Design review of the part built by this model. Coordinates are the model's own, in mm. Give positions to 0.01 mm unless a question says otherwise; leave off trailing zeros. Loops run counter-clockwise (first coordinate to the right, second up) from the corner with the lowest first, then second, coordinate; pieces in that order, holes last. Notation, with made-up numbers: (74, 71.25) -> (93, 71.25) arc R24 cw to (93, 101.25) -> close; hole circle Ø10 at (67.25, 40). An arc over 180 degrees is marked (long way). Answer as CSV lines item,"result".
from build123d import *

# Parameters (mm, degrees)
F1_DEPTH = 1.27
F2_DEPTH = 25.4


with BuildPart() as f1:
    # F0 (on Top) → F1 (new body)
    with BuildSketch(Plane.XY):
        with BuildLine():
            Line((-7.8964941204, 0.594703597), (-7.8964941204, -9.457487613))
            Line((-7.8964941204, -9.457487613), (-2.4395394139, -9.457487613))
            Line((-2.4395394139, -9.457487613), (-2.4395394139, 28.4462347627))
            Line((-2.4395394139, 28.4462347627), (0, 28.4462347627))
            Line((0, 28.4462347627), (0, -9.457487613))
            Line((0, -9.457487613), (7.2978408041, -9.457487613))
            Line((7.2978408041, -9.457487613), (7.2978408041, 0.594703597))
            Line((7.2978408041, 0.594703597), (4.625886213, 7.7879833989))
            Line((4.625886213, 7.7879833989), (7.2978408041, 14.9506824091))
            Line((7.2978408041, 14.9506824091), (4.6798829606, 19.9893178358))
            Line((4.6798829606, 19.9893178358), (4.410501927, 20.5077802788))
            Line((4.410501927, 20.5077802788), (5.1833918382, 21.9942174312))
            Line((5.1833918382, 21.9942174312), (7.2978408041, 26.0607674718))
            ThreePointArc((7.2978408041, 26.0607674718), (4.591156401, 30.2353352308), (7.2978408041, 34.4099029899))
            Line((7.2978408041, 34.4099029899), (-7.8964941204, 34.4099029899))
            ThreePointArc((-7.8964941204, 34.4099029899), (-5.1649912395, 30.2353352308), (-7.8964941204, 26.0607674718))
            Line((-7.8964941204, 26.0607674718), (-5.7663979357, 21.9942174312))
            Line((-5.7663979357, 21.9942174312), (-6.2874402602, 20.992138535))
            Line((-6.2874402602, 20.992138535), (-5.7663979357, 19.9893178358))
            Line((-5.7663979357, 19.9893178358), (-7.8964941204, 14.9506824091))
            Line((-7.8964941204, 14.9506824091), (-5.2315704525, 7.7879833989))
            Line((-5.2315704525, 7.7879833989), (-7.8964941204, 0.594703597))
        make_face()
        Polygon((0, 44.3628914654), (-7.8964941204, 34.4099029899), (7.2978408041, 34.4099029899), align=None)
    extrude(amount=F1_DEPTH)

    # F2 (add): faces of the model
    f2_faces = [f1.faces().sort_by_distance(p)[0] for p in [
        (-5.1680167671, -9.457487613, 0.635),
        (3.648920402, -9.457487613, 0.635),
    ]]
    extrude(f2_faces, amount=F2_DEPTH)


solid = f1.part
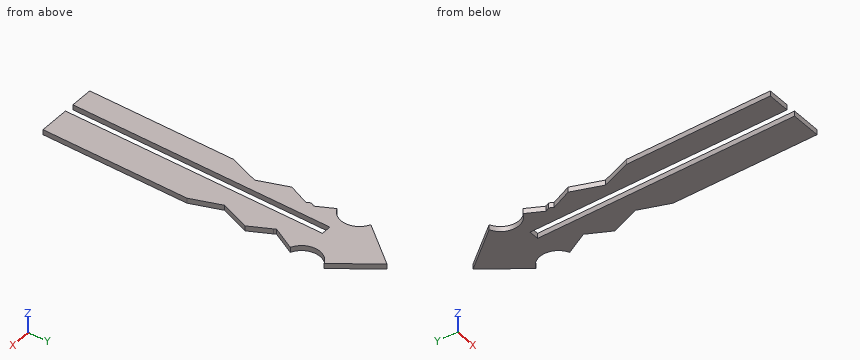
Q1. We need section D-D, the plane x = -3.25. State the section outline as (y, z) points, and give its area (3 significant figures).
Filled sheet:
outline,"(-34.86, 0) -> (40.27, 0) -> (40.27, 1.27) -> (-34.86, 1.27) -> close"
area,"95.4 mm^2"
Q2. We need section B-B, the plane z = 0.7. State the section outline as (x, y) points, and give its area (3 significant figures).
Filled sheet:
outline,"(-7.9, -34.86) -> (-2.44, -34.86) -> (-2.44, 28.45) -> (0, 28.45) -> (0, -34.86) -> (7.3, -34.86) -> (7.3, 0.59) -> (4.63, 7.79) -> (7.3, 14.95) -> (4.41, 20.51) -> (7.3, 26.06) arc R4.57 cw to (7.3, 34.41) -> (0, 44.36) -> (-7.9, 34.41) arc R4.56 cw to (-7.9, 26.06) -> (-5.77, 21.99) -> (-6.29, 20.99) -> (-5.77, 19.99) -> (-7.9, 14.95) -> (-5.23, 7.79) -> (-7.9, 0.59) -> close"
area,"873 mm^2"
Q3. We need section C-C, the plane y = 18. State the section outline as (x, z) points.
Filled sheet:
outline,"(-6.61, 0) -> (-2.44, 0) -> (-2.44, 1.27) -> (-6.61, 1.27) -> close; (0, 0) -> (5.71, 0) -> (5.71, 1.27) -> (0, 1.27) -> close"
Q4. We need section A-A, the plane y = 7. State the section outline as (x, z) points, and give its area (3 significant figures).
Filled sheet:
outline,"(-5.52, 0) -> (-2.44, 0) -> (-2.44, 1.27) -> (-5.52, 1.27) -> close; (0, 0) -> (4.92, 0) -> (4.92, 1.27) -> (0, 1.27) -> close"
area,"10.2 mm^2"
Q5. To check wall thickness, follow probe 1 along X at (y, z) = (-3.5, 1); probe 2 along X at (y, z) = (21, 0.55); probe 3 along X at (y, z) = (34.5, 0.3). State the ranges of each line that lie inside material, in increasing order. Write a range as from..to.
Filled sheet:
probe 1,"x = -7.9..-2.44, 0..7.3"
probe 2,"x = -6.28..-2.44, 0..4.67"
probe 3,"x = -7.83..7.23"
